CAD build for the part. Positions are in the model's coordinates, mm. Face numbers are marked on the shaded views. A direction names the side the tool comes from. Round coordinates to 2 decimals unless told otherwise and drop trailing zeros. Loops run counter-clockwise (first coordinate to the right, second up) from the corner with the lowest first, then second, coordinate; pieces in that order, holes last. Notation, with made-up numbers: (13, 54.25) - (26, 54.25) arc R22 cw to (26, 67.25) - close; hole circle Ø4 at (56.5, 16). An arc over 180 degrees is marked (long way). One line per question, with ' | ' between items.
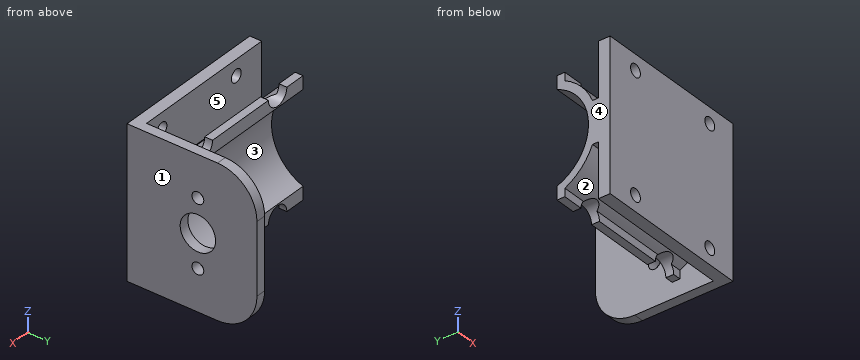
Autodesk Inventor part; units mm, degrees
ref_plane "YZ Plane" through (0, 0, 0) normal (1, 0, 0) x (0, 1, 0)
ref_plane "XZ Plane" through (0, 0, 0) normal (0, 1, 0) x (-1, 0, 0)
ref_plane "XY Plane" through (0, 0, 0) normal (0, 0, 1) x (1, 0, 0)
sketch "Boceto1" plane through (0, 0, 0) normal (0, 1, 0) x (-1, 0, 0)
  point P0 (0, 0)
sketch "Boceto2" plane through (0, 0, 0) normal (0, 1, 0) x (-1, 0, 0)
  line L0 (0, 0) -> (40, 0)
  line L1 (40, 0) -> (40, -38)
  line L2 (40, -38) -> (0, -38)
  line L3 (0, -38) -> (0, 0)
  dimension "d0" = 40
  dimension "d1" = 38
extrude "Extrusión1" add sketch "Boceto2" along normal blind 3
sketch "Boceto3" plane through (0, 3, 0) normal (0, 1, 0) x (1, 0, 0)
  line L0 (0, 0) -> (0, 38)
  line L1 (0, 0) -> (-2.5, 0)
  line L2 (-40, 0) -> (0, 0)
  line L3 (-2.5, 0) -> (-2.5, 38)
  line L4 (-2.5, 38) -> (0, 38)
  line L5 (0, 38) -> (0, 0)
  dimension "d4" = 2.5
  dimension "d5" = 38
extrude "Extrusión2" add sketch "Boceto3" along normal blind 30
sketch "Boceto4" plane through (0, 0, 0) normal (1, 0, 0) x (0, 0, -1)
  line L0 (0, 0) -> (38, 0)
  circle A0 centre (19, 18) radius 4.5
  line L1 (19, 0) -> (19, 18)
  dimension "d9" = 9
  dimension "d21" = 18
extrude "Extrusión3" cut sketch "Boceto4" against normal blind 30
sketch "Boceto5" plane through (0, 0, 0) normal (1, 0, 0) x (0, 0, -1)
  circle A0 centre (19, 18) radius 4.5
  line L0 (19, 18) -> (27.5, 18)
  line L1 (19, 18) -> (10.5, 18)
  circle A1 centre (10.5, 18) radius 1.5
  circle A2 centre (27.5, 18) radius 1.5
  point P0 (0, 0)
  dimension "d12" = 8.5
  dimension "d13" = 8.5
  dimension "d14" = 3
  dimension "d15" = 3
extrude "Extrusión4" cut sketch "Boceto5" against normal blind 8.5 contours A1 | A2
fillet "Empalme1" radius 10 1 edges at (-1.25, 33, 0)
fillet "Empalme2" radius 10 1 edges at (-1.25, 33, -38)
sketch "Boceto6" plane through (-2.5, 3, -38) normal (-1, 0, 0) x (0, 0, 1)
  circle A0 centre (19, 15) radius 4.5
  arc A1 (7.3381, 10.5) -> (30.6619, 10.5) centre (19, 15) ccw
  line L0 (30.6619, 10.5) -> (34, 10.5)
  circle A2 centre (19, 15) radius 4.5
  line L1 (4, 10.5) -> (7.3381, 10.5)
  line L2 (34, 8.5) -> (31.9615, 8.5)
  arc A3 (6.0385, 8.5) -> (31.9615, 8.5) centre (19, 15) ccw
  line L3 (6.0385, 8.5) -> (4, 8.5)
  line L4 (4, 10.5) -> (4, 8.5)
  line L5 (0, 0) -> (0, 20)
  line L6 (34, 10.5) -> (34, 8.5)
  line L7 (38, 0) -> (38, 20)
  point P0 (38, -3)
  dimension "d20" = 25
  dimension "d27" = 2
extrude "Extrusión5" add sketch "Boceto6" along normal blind 37.5 contours A1 L0 L6 L2 A3 L3 L4 L1
sketch "Boceto9" plane through (0, 0, 0) normal (0, -1, 0) x (1, 0, 0)
  line L0 (0, 0) -> (0, -38)
  line L1 (0, -38) -> (0, -19)
  line L2 (0, -19) -> (-7.55, -19)
  line L3 (-7.55, -19) -> (-7.55, -4)
  line L4 (-7.55, -19) -> (-7.55, -34)
  circle A0 centre (-7.55, -4) radius 1.6
  circle A1 centre (-7.55, -34) radius 1.6
  line L5 (-7.55, -4) -> (-31.75, -4)
  line L6 (-2.5, -4) -> (-40, -4)
  line L7 (-31.75, -4) -> (-31.75, -34)
  circle A2 centre (-31.75, -4) radius 1.6
  circle A3 centre (-31.75, -34) radius 1.6
  dimension "d33" = 19
  dimension "d34" = 7.55
  dimension "d35" = 15
  dimension "d37" = 15
  dimension "d38" = 3.2
  dimension "d39" = 3.2
  dimension "d41" = 24.2
  dimension "d42" = 30
  dimension "d43" = 3.2
  dimension "d44" = 3.2
extrude "Extrusión6" cut sketch "Boceto9" against normal blind 3
sketch "Boceto10" plane through (0, 3, 0) normal (0, 1, 0) x (1, 0, 0)
  circle A0 centre (-31.75, 4) radius 1.6
  circle A1 centre (-31.75, 4) radius 3
  circle A2 centre (-7.55, 4) radius 1.6
  circle A3 centre (-7.55, 4) radius 3
  circle A4 centre (-31.75, 34) radius 1.6
  circle A5 centre (-31.75, 34) radius 3
  line L0 (-2.5, 34) -> (-40, 34)
  circle A6 centre (-7.55, 34) radius 3
  point P0 (0, 0)
  dimension "d58" = 6
  dimension "d59" = 6
  dimension "d60" = 6
  dimension "d61" = 6
extrude "Extrusión7" cut sketch "Boceto10" along normal blind 20 contours A0 | A1 | A2 | A3 | L0 A4 | L0 A5 A4 | A4 L0 A5 | A4 L0 | A6 L0 | L0 A6
sketch "Boceto11" plane through (-40, 0, -38) normal (-1, 0, 0) x (0, 0, 1)
  line L0 (0, 3) -> (38, 3)
  arc A0 (6.0385, 11.5) -> (31.9615, 11.5) centre (19, 18) ccw
  line L1 (19, 4.5) -> (24.2915, 4.5)
  line L2 (19, 4.5) -> (13.7085, 4.5)
  line L3 (13.7085, 4.5) -> (13.7085, 3)
  line L4 (24.2915, 4.5) -> (24.2915, 3)
  line L5 (13.7085, 3) -> (24.2915, 3)
  point P0 (38, 0)
extrude "Extrusión8" add sketch "Boceto11" against normal blind 40
equation "\"d16\" = d12"
equation "\"Radio_pliegue\" = Grosor"
equation "\"Anchura_desahogo_plegado\" = Grosor"
equation "\"Profundidad_desahogo_plegado\" = 0.5 * Grosor"
equation "\"Tamaño_destalonado\" = 4 * Grosor"
equation "\"Remanente_mínimo\" = 2 * Grosor"
equation "\"Radiodetransición\" = Radio_pliegue"
equation "\"Tamaño_de_radio_de_Jacobi\" = Radio_pliegue"
equation "\"TamañoSeparación\" = Grosor"
properties part number "Base_nueva_3DPrint"
(1) Tool access for the marked faces 1 and 2: list every direction of +Z, -Z, +X, -X, +Y, -Y with a clear straight run to the whole face (end or side of a thin tool).
Results found:
face 1: +Z, -Z, +X, +Y, -Y | face 2: -Z, -X
(2) Cut at A-A, the plane y = 18. Write the cut outline in (x, z).
Results found:
outline: (-2.5, -38) - (0, -38) - (0, -29) - (-2.5, -29) - close; (-2.5, -26) - (0, -26) - (0, -23.5) - (-2.5, -23.5) - close; (-2.5, -14.5) - (0, -14.5) - (0, -12) - (-2.5, -12) - close; (-2.5, -9) - (0, -9) - (0, 0) - (-2.5, 0) - close
(3) Cut at B-B, the plane x = -31.75. Write the cut outline in (y, z).
Results found:
outline: (0, -38) - (3, -38) - (3, -35.6) - (0, -35.6) - close; (0, -32.4) - (3, -32.4) - (3, -24.29) - (4.5, -24.29) arc R14.5 ccw to (9.86, -31) - (13.5, -31) - (13.5, -30.66) arc R12.5 cw to (13.5, -7.34) - (13.5, -7) - (9.86, -7) arc R14.5 ccw to (4.5, -13.71) - (3, -13.71) - (3, -5.6) - (0, -5.6) - close; (0, -2.4) - (3, -2.4) - (3, 0) - (0, 0) - close
(4) Probe L1, parallel to Z at x = -31.75, y = 0.65; L2, parallel to Y at x = -1.25, z = -27.5; L3, parallel to Z at x = -7, y = 1. List the from-to ranges inside material, lowest first.
Results found:
L1: z = -38 to -35.6, -32.4 to -5.6, -2.4 to 0 | L2: y = 0 to 16.5, 19.5 to 33 | L3: z = -38 to -35.5, -32.5 to -5.5, -2.5 to 0
(5) Cut at D-D, the plane x = -14. Write the cut outline in (y, z), then the cut area to 3 significant figures.
Results found:
outline: (0, -38) - (3, -38) - (3, -24.29) - (4.5, -24.29) arc R14.5 ccw to (11.5, -31.96) - (11.5, -34) - (13.5, -34) - (13.5, -30.66) arc R12.5 cw to (13.5, -7.34) - (13.5, -4) - (11.5, -4) - (11.5, -6.04) arc R14.5 ccw to (4.5, -13.71) - (3, -13.71) - (3, 0) - (0, 0) - close | area: 196 mm²
(6) Two-plate mould, pull along Y, no slides. Class the marked faces 3, 4 and 5: released by +Y, released by -Y, zero draft, split by the parting line, or undercut.
Results found:
face 3: released by +Y | face 4: zero draft | face 5: undercut
(7) Drop flat-ended pins along their axis: P1, Ø5, axis at x = -19.5, z = -17.5, coming from the +Y side; P2, Ø11, axis at x = -27, z = -30.5, coming from the +Y side; P3, Ø1, axis at x = -37.5, y = 12.5, coming from the +Z side. Give the stop position or say it passes through.
Results found:
P1: stops at y = 6.16 | P2: stops at y = 13.5 | P3: stops at z = -4
(8) Cut at C-C, the plane z = -19. Write the cut outline in (x, y), then the cut area to 3 significant figures.
Results found:
outline: (-40, 0) - (0, 0) - (0, 13.5) - (-2.5, 13.5) - (-2.5, 5.5) - (-40, 5.5) - close; (-2.5, 22.5) - (0, 22.5) - (0, 33) - (-2.5, 33) - close | area: 266 mm²
